Source: CAD feature listing. Evaluate the final solid. Frame: model axes, mm. A direction names the side the tool comes from. Round coordinates to 2 decimals unless told otherwise and drop trailing zeros. Write each loop counter-clockwise with the first axis right and the second up, starting at its lowest first coordinate (ties: lowest second). Pieces come first, ordered by that corner, then holes. Notation, with made-up numbers: M 73.25,-30 L 124.25,-30 A30 cw 124.25,-2 Z; hole C -8,34 d5. An arc over 180 degrees is marked long. Answer in a Markdown table with one row per item.
from build123d import *

# Parameters (mm, degrees)
F0_R        = 11.938
F1_DEPTH    = 15.24
F0_R_2      = 6.7437
F2_DEPTH    = 14.224
F5_DEPTH    = 45.72
F6_T1_DEPTH = 147.32
F6_T3_DEPTH = 147.32


# Not quite as in the source:
# - a fillet or chamfer that OpenCascade refuses, or shapes differently, is made with other operations: its cross-section is extruded or revolved along the edge and cut away or added


with BuildPart() as f1:
    # F0 (on Top) → F1 (new body)
    with BuildSketch(Plane.XY):
        with BuildLine():
            ThreePointArc((44.45, -25.4), (69.85, 0), (44.45, 25.4))
            Line((44.45, 25.4), (-44.45, 25.4))
            ThreePointArc((-44.45, 25.4), (-69.85, 0), (-44.45, -25.4))
            Line((-44.45, -25.4), (44.45, -25.4))
        make_face()
        with Locations((-44.45, 0)):
            Circle(F0_R, mode=Mode.SUBTRACT)
        with Locations((44.45, 0)):
            Circle(F0_R, mode=Mode.SUBTRACT)
    extrude(amount=F1_DEPTH)

    # F0 (on Top) → F2 (join)
    with BuildSketch(Plane.XY):
        with Locations((-44.45, 0)):
            Circle(F0_R)
        with Locations((-44.45, 0)):
            Circle(F0_R_2, mode=Mode.SUBTRACT)
        with Locations((44.45, 0)):
            Circle(F0_R)
        with Locations((44.45, 0)):
            Circle(F0_R_2, mode=Mode.SUBTRACT)
    extrude(amount=F2_DEPTH)

    # F4 (on face) → F5 (join)
    with BuildSketch(Plane.XY.offset(15.24)):
        Polygon((-25.7984097937, -11.0315902063), (-11.43, -25.4), (20.8989220358, 6.9289220358), (6.5305122421, 21.2973318296), align=None)
    extrude(amount=F5_DEPTH)

    # F6: fillet of radius 25.4 on 2 edges, made by hand

    # F6_s2 → F6_t1 (cut)
    with BuildSketch(Plane(origin=(-52.2846903991, 52.2846903991, 0), x_dir=(0, 0, 1), z_dir=(0.7071067812, -0.7071067812, 0))):
        with BuildLine():
            ThreePointArc((35.56, 26.0427427511), (53.5205122421, 18.6032549932), (60.96, 0.6427427511))
            Line((60.96, 0.6427427511), (60.96, 26.0427427511))
            Line((60.96, 26.0427427511), (35.56, 26.0427427511))
        make_face()
    extrude(amount=F6_T1_DEPTH, mode=Mode.SUBTRACT)

    # F6_s4 → F6_t3 (cut)
    with BuildSketch(Plane(origin=(51.8862806053, -51.8862806053, 0), x_dir=(0, 0, 1), z_dir=(-0.7071067812, 0.7071067812, 0))):
        with BuildLine():
            ThreePointArc((35.56, 19.6772572489), (53.5205122421, 12.237769491), (60.96, -5.7227427511))
            Line((60.96, -5.7227427511), (60.96, 19.6772572489))
            Line((60.96, 19.6772572489), (35.56, 19.6772572489))
        make_face()
    extrude(amount=F6_T3_DEPTH, mode=Mode.SUBTRACT)


solid = f1.part
Q1. Section D-D (z = 55). Return loops of the section in (x, y).
Solutions:
| item | result |
|---|---|
| outline | M -19.4,-4.63 L -5.03,-19 L 14.5,0.53 L 0.13,14.9 Z |
Q2. Section A-A (z = 10). Return loops of the section in (x, y).
Solutions:
| item | result |
|---|---|
| outline | M -44.45,-25.4 L 44.45,-25.4 A25.4 ccw 44.45,25.4 L -44.45,25.4 A25.4 ccw Z; hole C -44.45,0 d13.49; hole C 44.45,0 d13.49 |
Q3. Pull-direction query (X, two-part tool) for faces 5 (the flat face through (-39, -5, 14.224)), 6 (the cylindrical face through (69.844, -0.559, 7.513)), 7 (the cylindrical face through (-14.2, -13.6, 52.4)); classes: pulls with the +X half, pulls with the -X half, needs draft (parallel to the pull), parting line crosses it, or undercut.
Solutions:
| item | result |
|---|---|
| face 5 | undercut |
| face 6 | pulls with the +X half |
| face 7 | pulls with the -X half |
Q4. Access query for faces 1 (the flat face through (-18.71, -18.12, 25.26)), 2 (the flat face through (13.82, 14.01, 25.26)), 3 (the flat face through (4.51, -9.46, 37.72)), 4 (the flat face through (15, 0, 15.24)). Directions: +Z, -Z, +X, -X, +Y, -Y. A direction counts if a zero-diameter tool reaches every point of the face in a straight line with its end or side. Return the directions, or none.
Solutions:
| item | result |
|---|---|
| face 1 | +Z, -X, -Y |
| face 2 | +Z, +X, +Y |
| face 3 | +Z, +X, -Y |
| face 4 | +Z |
Q5. Section B-B (y = 0). State how many separate pieces and enclosed holes the cut face has, and give its area (3 significant figures).
Solutions:
| item | result |
|---|---|
| separate pieces | 3 |
| enclosed holes | 0 |
| area | 2,960 mm2 |
Q6. Contact query for flat-ended pins moving along their axis: pin 1 Ø12 at (x, y) = (-44, -4) entering from +Z; pin 2 Ø19 at (x, y) = (39.5, -3.5) entering from +Z; pin 3 Ø5 at (y, z) = (-15.5, 16) entering from +X. Output: stop coordinate, or through.
Solutions:
| item | result |
|---|---|
| pin 1 | stops at z = 14.22 |
| pin 2 | stops at z = 15.24 |
| pin 3 | stops at x = 66.2 |
Q7. Material intervals for probe 1 along Y at (x, z) = (44.45, 14.8); probe 2 along Y at (x, z) = (44, 10); probe 3 along Z at (x, y) = (-0.5, -16.5), sorted ascending.
Solutions:
| item | result |
|---|---|
| probe 1 | y = -25.4 to -11.94, 11.94 to 25.4 |
| probe 2 | y = -25.4 to -6.73, 6.73 to 25.4 |
| probe 3 | z = 0 to 15.24 |
Q8. Section C-C (z = 28). Return loops of the section in (x, y).
Solutions:
| item | result |
|---|---|
| outline | M -25.8,-11.03 L -11.43,-25.4 L 20.9,6.93 L 6.53,21.3 Z |
